Model file for the job. Use its own axes, mm. Round coordinates to 2 decimals unless told otherwise and drop trailing zeros. Order: outer loops, then holes, each group sorted by start corner. A loop starts at its lowest first (then second) coordinate and runs counter-clockwise, first axis right, second up. Notation, with made-up numbers: (31.5, 80.25) -> (81.5, 80.25) arc R26 cw to (81.5, 108.25) -> close; hole circle Ø6 at (-7.5, 40.25). An arc over 180 degrees is marked (long way). Answer as CSV lines item,"result".
```python
from build123d import *

# Parameters (mm, degrees)
F0_R     = 1.27
F1_DEPTH = 64.77
F2_SIZE  = 1.27
F3_R     = 0.127
F4_DEPTH = 64.771


with BuildPart() as f1:
    # F0 (on Top) → F1 (new body)
    with BuildSketch(Plane.XY):
        Circle(F0_R)
    extrude(amount=F1_DEPTH)

    # F2
    f2_edges = [f1.edges().sort_by_distance(p)[0] for p in [
        (-1.27, 0, 64.77),
    ]]
    chamfer(f2_edges, length=F2_SIZE)

    # F3 (on face) → F4 (cut, through all)
    with BuildSketch(Plane(origin=(0, 0, 0), x_dir=(1, 0, 0), z_dir=(0, 0, -1))):
        Circle(F3_R)
    extrude(amount=-F4_DEPTH, mode=Mode.SUBTRACT)


solid = f1.part
```
Q1. Saw through at A-A (z = 20). Write the cut outline in (x, y), plus the area to 3 significant figures.
Checks:
outline,"circle Ø2.54 at (0, 0); hole circle Ø0.25 at (0, 0)"
area,"5.02 mm²"
Q2. Wall check: L1, parallel to Y at x = 0, z = 42.5; L2, parallel to Y at x = 0.25, z = 8.5. Give the ranges that are in metal, low to high. Write a range as [from, to].
Checks:
L1,"[-1.27, -0.13], [0.13, 1.27]"
L2,"[-1.25, 1.25]"
Q3. Mould opens along Y. For faces 1 (the cylindrical face through (-0.17, 1.26, 31.31)), 2 (the flat face through (0.3, 0, 0)) say: +Y half, -Y half, draft (parallel to the pull), parting line (faces both ways), or undercut.
Checks:
face 1,"parting line"
face 2,"draft"
Q4. Flat gauge pins, fed straight in: pin 1 (1.5 mm diameter, centred on x = 0.5, y = 0, fed in from -Z); pin 2 (1 mm diameter, centred on x = 0.5, y = 0.5, fed in from +Z). Where does each tip first touch, or does it go through?
Checks:
pin 1,"z = 0"
pin 2,"z = 64.56"
